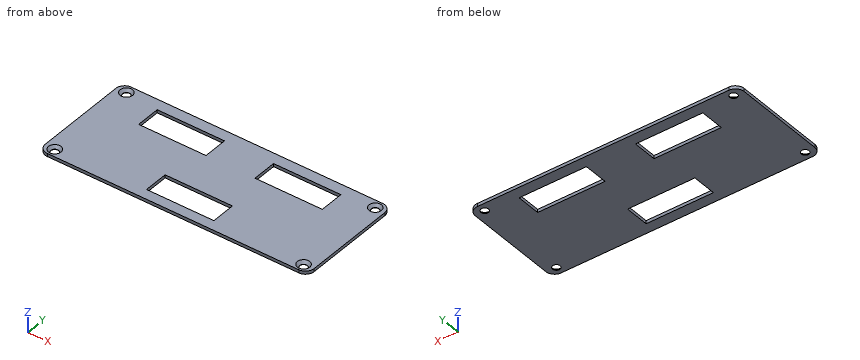
```python
from build123d import *

# Parameters (mm, degrees)
SKETCH1_W                                      = 124.8
SKETCH1_H                                      = 50.9
BOSS_EXTRUDE1_DEPTH                            = 1.45
CSK_FOR_M3_5_FLAT_HEAD_MACHINE_SCREW1_AT_COUNT = 2
CSK_FOR_M3_5_FLAT_HEAD_MACHINE_SCREW1_AT_PITCH = 115.5
CSK_FOR_M3_5_FLAT_HEAD_MACHINE_SCREW_2_COUNT   = 2
CSK_FOR_M3_5_FLAT_HEAD_MACHINE_SCREW_2_PITCH   = 123.420014584
CSK_FOR_M3_5_FLAT_HEAD_MACHINE_SCREW_3_COUNT   = 2
CSK_FOR_M3_5_FLAT_HEAD_MACHINE_SCREW_3_PITCH   = 43.5
FILLET2_R                                      = 4
SKETCH4_W                                      = 31.25
SKETCH4_H                                      = 11.25
CUT_EXTRUDE1_DEPTH                             = 1.45


with BuildPart() as part:
    # Sketch1 → Boss-Extrude1 (new body)
    with BuildSketch(Plane.XY):
        with Locations((62.4, -25.45)):
            Rectangle(SKETCH1_W, SKETCH1_H)
    extrude(amount=BOSS_EXTRUDE1_DEPTH)

    # Sketch2 → CSK for M3.5 Flat Head Machine Screw1 (revolve, cut)
    with BuildSketch(Plane(origin=(4.65, -3.7, 1.45), x_dir=(0, -1, 0), z_dir=(1, 0, 0))):
        Polygon((0, 0), (0, 1.45), (1.75, 1.45), (1.75, 1.294164458), (2.875, 0), align=None)
    csk_for_m3_5_flat_head_machine_screw1 = revolve(axis=Axis((4.65, -3.7, 7.8), (0, 0, -1)), mode=Mode.SUBTRACT)

    # CSK for M3.5 Flat Head Machine Screw1 at: CSK for M3.5 Flat Head Machine Screw1 ×2
    with Locations(*[(i * CSK_FOR_M3_5_FLAT_HEAD_MACHINE_SCREW1_AT_PITCH, 0, 0) for i in range(1, CSK_FOR_M3_5_FLAT_HEAD_MACHINE_SCREW1_AT_COUNT)]):
        add(csk_for_m3_5_flat_head_machine_screw1, mode=Mode.SUBTRACT)

    # CSK for M3.5 Flat Head Machine Screw 2: CSK for M3.5 Flat Head Machine Screw1 ×2
    with Locations(*[Vector(0.935828766, -0.35245499, 0) * (i * CSK_FOR_M3_5_FLAT_HEAD_MACHINE_SCREW_2_PITCH) for i in range(1, CSK_FOR_M3_5_FLAT_HEAD_MACHINE_SCREW_2_COUNT)]):
        add(csk_for_m3_5_flat_head_machine_screw1, mode=Mode.SUBTRACT)

    # CSK for M3.5 Flat Head Machine Screw 3: CSK for M3.5 Flat Head Machine Screw1 ×2
    with Locations(*[(0, -i * CSK_FOR_M3_5_FLAT_HEAD_MACHINE_SCREW_3_PITCH, 0) for i in range(1, CSK_FOR_M3_5_FLAT_HEAD_MACHINE_SCREW_3_COUNT)]):
        add(csk_for_m3_5_flat_head_machine_screw1, mode=Mode.SUBTRACT)

    # Fillet2
    fillet2_edges = [part.edges().sort_by_distance(p)[0] for p in [
        (0, 0, 0.725),
        (124.8, 0, 0.725),
        (124.8, -50.9, 0.725),
        (0, -50.9, 0.725),
    ]]
    fillet(fillet2_edges, radius=FILLET2_R)

    # Sketch4 → Cut-Extrude1 (cut)
    with BuildSketch(Plane.XY):
        with Locations((35.651, -10.75)):
            Rectangle(SKETCH4_W, SKETCH4_H)
        with Locations((89.651, -10.75)):
            Rectangle(SKETCH4_W, SKETCH4_H)
        with Locations((62.069, -40.5)):
            Rectangle(SKETCH4_W, SKETCH4_H)
    extrude(amount=CUT_EXTRUDE1_DEPTH, mode=Mode.SUBTRACT)


solid = part.part
```
Build history of the part. All positions in model axes, mm. Round coordinates to 2 decimals unless told otherwise and drop trailing zeros. Write each loop counter-clockwise with the first axis right and the second up, starting at its lowest first coordinate (ties: lowest second). Pieces come first, ordered by that corner, then holes.
1) Band-saw the part on B-B, the plane x = 101. List the corners of the cut face in (y, z) (3 decimals).
2) Band-saw the part on C-C, the plane z = 0.8. List the corners of the cut face in (x, y) (3 decimals).
3) Drill centre lines: probe 1 along Y at (x, z) = (4.65, 0.1); probe 2 along X at (y, z) = (-3.7, 0.1); probe 3 along Y at (x, z) = (91, 0.2) (3 decimals). Where is each one in solid material? Low to high.
4) Pin check, flat tip, straight feed: pin 1 (2 mm diameter, centred on x = 4.65, y = -3.7, fed in from +Z) (3 decimals). Stop position of the tip, or through.
5) Band-saw the part on A-A, the plane y = -38. List the corners of the cut face in (x, z).
Ans:
1. outline: (-50.9, 0) - (-16.375, 0) - (-16.375, 1.45) - (-50.9, 1.45) - close; (-5.125, 0) - (0, 0) - (0, 1.45) - (-5.125, 1.45) - close
2. outline: (0, -46.9) arc R4 ccw to (4, -50.9) - (120.8, -50.9) arc R4 ccw to (124.8, -46.9) - (124.8, -4) arc R4 ccw to (120.8, 0) - (4, 0) arc R4 ccw to (0, -4) - close; hole circle Ø4.62 at (4.65, -47.2); hole circle Ø4.62 at (4.65, -3.7); hole (20.026, -16.375) - (51.276, -16.375) - (51.276, -5.125) - (20.026, -5.125) - close; hole (46.444, -46.125) - (77.694, -46.125) - (77.694, -34.875) - (46.444, -34.875) - close; hole (74.026, -16.375) - (105.276, -16.375) - (105.276, -5.125) - (74.026, -5.125) - close; hole circle Ø4.62 at (120.15, -47.2); hole circle Ø4.62 at (120.15, -3.7)
3. probe 1: y = -50.9 to -48.95, -45.45 to -5.45, -1.95 to 0
3. probe 2: x = 0.01 to 2.9, 6.4 to 118.4, 121.9 to 124.79
3. probe 3: y = -50.9 to -16.375, -5.125 to 0
4. pin 1: passes through
5. outline: (0, 0) - (46.44, 0) - (46.44, 1.45) - (0, 1.45) - close; (77.69, 0) - (124.8, 0) - (124.8, 1.45) - (77.69, 1.45) - close
